The listing builds one solid part. Answer for the finished solid, in the listing's coordinates (mm). Give positions to 0.01 mm unless a question says otherwise; leave off trailing zeros. Loops run counter-clockwise (first coordinate to the right, second up) from the corner with the lowest first, then second, coordinate; pieces in that order, holes last. Notation, with made-up numbers: M 88.5,-31 L 98.5,-31 A15 ccw 98.5,-14 Z; hole C 19,-17.75 d2. An arc over 180 degrees is marked long. Use one line per item in the form item = value. Start each with the question number.
1. The part is cut by section C-C (y = 10). Write down the section's boundary in (x, z).
2. Straight lines are drawn through the part: line 1 (X direction, y = 23.5, z = 0.85); line 2 (Y direction, x = 9.5, z = 0.6) (3 decimals); line 3 (X direction, y = 23, z = 0.3). For each, find the intervals that lie inside material, in ascending order. Write a range as from..to.
3. The part is cut by section D-D (x = 21). Write down the section's boundary in (y, z).
4. The part is cut by section A-A (y = 4). Write down the section's boundary in (x, z), and give its area (3 significant figures).
5. The part is cut by section B-B (x = 26). Write down the section's boundary in (y, z), and give its area (3 significant figures).
6. Each of these flat-tipped pins is pushed along its axis until it touches: pin 1 Ø1.6 at (x, y) = (7.99, 38.71) entering from -Z; pin 2 Ø8 at (x, y) = (5, 13) entering from -Z. Where does it stop, or does it pass through?
from build123d import *

# Parameters (mm, degrees)
MODEL_W             = 35.3822
MODEL_H             = 41.1734
MODEL_R             = 0.97623725
MODEL_R_2           = 0.9398
MODEL_R_3           = 2.1079968
MODEL_R_4           = 0.889
MODEL_W_2           = 7.62
MODEL_H_2           = 19.05
MODEL_W_3           = 8.89
MODEL_H_3           = 10.16
BOSS_EXTRUDE3_DEPTH = 2.54


with BuildPart() as part:
    # Model → Boss-Extrude3 (new body)
    with BuildSketch(Plane.XY):
        with Locations((17.6911, 20.5867)):
            Rectangle(MODEL_W, MODEL_H)
        with Locations((19.05, 12.065)):
            Circle(MODEL_R, mode=Mode.SUBTRACT)
        with Locations((19.05, 14.605)):
            Circle(MODEL_R_2, mode=Mode.SUBTRACT)
        with Locations((19.05, 26.035)):
            Circle(MODEL_R_2, mode=Mode.SUBTRACT)
        with Locations((19.05, 23.495)):
            Circle(MODEL_R_2, mode=Mode.SUBTRACT)
        with Locations((19.05, 20.955)):
            Circle(MODEL_R_2, mode=Mode.SUBTRACT)
        with Locations((26.4033, 3.175)):
            Circle(MODEL_R_3, mode=Mode.SUBTRACT)
        with Locations((2.9083, 38.7096)):
            Circle(MODEL_R_4, mode=Mode.SUBTRACT)
        with Locations((2.9083, 36.1696)):
            Circle(MODEL_R_4, mode=Mode.SUBTRACT)
        with Locations((5.4483, 36.1696)):
            Circle(MODEL_R_4, mode=Mode.SUBTRACT)
        with Locations((7.9883, 36.1696)):
            Circle(MODEL_R_4, mode=Mode.SUBTRACT)
        with Locations((10.5283, 36.1696)):
            Circle(MODEL_R_4, mode=Mode.SUBTRACT)
        with Locations((13.0683, 36.1696)):
            Circle(MODEL_R_4, mode=Mode.SUBTRACT)
        with Locations((5.4483, 38.7096)):
            Circle(MODEL_R_4, mode=Mode.SUBTRACT)
        with Locations((7.9883, 38.7096)):
            Circle(MODEL_R_4, mode=Mode.SUBTRACT)
        with Locations((10.5283, 38.7096)):
            Circle(MODEL_R_4, mode=Mode.SUBTRACT)
        with Locations((13.0683, 38.7096)):
            Circle(MODEL_R_4, mode=Mode.SUBTRACT)
        with Locations((15.6083, 38.7096)):
            Circle(MODEL_R_4, mode=Mode.SUBTRACT)
        with Locations((15.6083, 36.1696)):
            Circle(MODEL_R_4, mode=Mode.SUBTRACT)
        with Locations((18.1483, 36.1696)):
            Circle(MODEL_R_4, mode=Mode.SUBTRACT)
        with Locations((20.6883, 36.1696)):
            Circle(MODEL_R_4, mode=Mode.SUBTRACT)
        with Locations((23.2283, 36.1696)):
            Circle(MODEL_R_4, mode=Mode.SUBTRACT)
        with Locations((25.7683, 36.1696)):
            Circle(MODEL_R_4, mode=Mode.SUBTRACT)
        with Locations((18.1483, 38.7096)):
            Circle(MODEL_R_4, mode=Mode.SUBTRACT)
        with Locations((20.6883, 38.7096)):
            Circle(MODEL_R_4, mode=Mode.SUBTRACT)
        with Locations((23.2283, 38.7096)):
            Circle(MODEL_R_4, mode=Mode.SUBTRACT)
        with Locations((25.7683, 38.7096)):
            Circle(MODEL_R_4, mode=Mode.SUBTRACT)
        with Locations((28.3083, 38.7096)):
            Circle(MODEL_R_4, mode=Mode.SUBTRACT)
        with Locations((28.3083, 36.1696)):
            Circle(MODEL_R_4, mode=Mode.SUBTRACT)
        with Locations((30.8483, 36.1696)):
            Circle(MODEL_R_4, mode=Mode.SUBTRACT)
        with Locations((33.3883, 36.1696)):
            Circle(MODEL_R_4, mode=Mode.SUBTRACT)
        with Locations((30.8483, 38.7096)):
            Circle(MODEL_R_4, mode=Mode.SUBTRACT)
        with Locations((33.3883, 38.7096)):
            Circle(MODEL_R_4, mode=Mode.SUBTRACT)
        with Locations((19.05, 9.525)):
            Circle(MODEL_R, mode=Mode.SUBTRACT)
        with Locations((19.05, 28.575)):
            Circle(MODEL_R, mode=Mode.SUBTRACT)
        with Locations((11.43, 20.32)):
            Rectangle(MODEL_W_2, MODEL_H_2, mode=Mode.SUBTRACT)
        with Locations((27.305, 11.43)):
            Rectangle(MODEL_W_3, MODEL_H_3, mode=Mode.SUBTRACT)
    extrude(amount=BOSS_EXTRUDE3_DEPTH)


solid = part.part
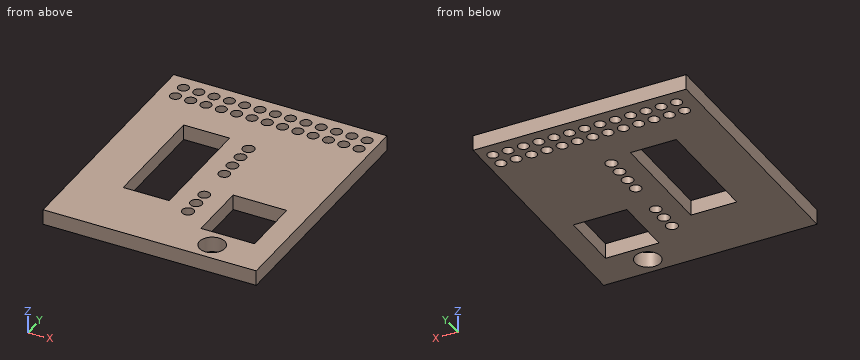
Derived:
q1.outline = M 0,0 L 18.2,0 L 18.2,2.54 L 0,2.54 Z; M 19.9,0 L 22.86,0 L 22.86,2.54 L 19.9,2.54 Z; M 31.75,0 L 35.38,0 L 35.38,2.54 L 31.75,2.54 Z
q2.line_1 = 0..7.62, 15.24..18.11, 19.99..35.38
q2.line_2 = 0..10.795, 29.845..41.173
q2.line_3 = 0..7.62, 15.24..18.25, 19.85..35.38
q3.outline = M 0,0 L 35.34,0 L 35.34,2.54 L 0,2.54 Z; M 37,0 L 37.88,0 L 37.88,2.54 L 37,2.54 Z; M 39.54,0 L 41.17,0 L 41.17,2.54 L 39.54,2.54 Z
q4.outline = M 0,0 L 24.46,0 L 24.46,2.54 L 0,2.54 Z; M 28.34,0 L 35.38,0 L 35.38,2.54 L 28.34,2.54 Z
q4.area = 80.0 mm2
q5.outline = M 0,0 L 1.11,0 L 1.11,2.54 L 0,2.54 Z; M 5.24,0 L 6.35,0 L 6.35,2.54 L 5.24,2.54 Z; M 16.51,0 L 35.31,0 L 35.31,2.54 L 16.51,2.54 Z; M 37.03,0 L 37.85,0 L 37.85,2.54 L 37.03,2.54 Z; M 39.57,0 L 41.17,0 L 41.17,2.54 L 39.57,2.54 Z
q5.area = 59.5 mm2
q6.pin_1 = through
q6.pin_2 = 0
